Build history of the part. All positions in model axes, mm. A direction names the side the tool comes from. Round coordinates to 2 decimals unless told otherwise and drop trailing zeros. Write each loop counter-clockwise with the first axis right and the second up, starting at its lowest first coordinate (ties: lowest second). Pieces come first, ordered by that corner, then holes.
from build123d import *

# Parameters (mm, degrees)
SKETCH_1_R          = 6
EXTRUDE_1_DEPTH     = 40
CUT_EXTRUDE_START   = -5
CUT_EXTRUDE_1_DEPTH = 5
CUT_EXTRUDE_2_DEPTH = 5


with BuildPart() as part:
    # 草图1 → 凸台-拉伸1 (new body)
    with BuildSketch(Plane.XY):
        Circle(SKETCH_1_R)
    extrude(amount=EXTRUDE_1_DEPTH)

    # 草图2 → 切除-拉伸1 (cut)
    with BuildSketch(Plane.XY.offset(40).offset(CUT_EXTRUDE_START)):
        with BuildLine():
            Line((2.5, 3), (-2.5, 3))
            Line((-2.5, 3), (-2.5, 5.454356057))
            ThreePointArc((-2.5, 5.454356057), (0, 6), (2.5, 5.454356057))
            Line((2.5, 5.454356057), (2.5, 3))
        make_face()
    extrude(amount=CUT_EXTRUDE_1_DEPTH, mode=Mode.SUBTRACT)

    # 草图3 → 切除-拉伸2 (cut)
    with BuildSketch(Plane(origin=(0, 0, 0), x_dir=(-1, 0, 0), z_dir=(0, 0, -1))):
        with BuildLine():
            Line((2.5, 3), (-2.5, 3))
            Line((-2.5, 3), (-2.5, 5.454356057))
            ThreePointArc((-2.5, 5.454356057), (0, 6), (2.5, 5.454356057))
            Line((2.5, 5.454356057), (2.5, 3))
        make_face()
    extrude(amount=-CUT_EXTRUDE_2_DEPTH, mode=Mode.SUBTRACT)


solid = part.part
1) Slice it at C-C (x = 1.75). Write the cut outline in (y, z).
Results:
outline: (-5.74, 0) - (3, 0) - (3, 5) - (5.74, 5) - (5.74, 35) - (3, 35) - (3, 40) - (-5.74, 40) - close
2) Slice it at B-B (z = 12). Write the cut outline in (x, y), plus the area to 3 significant figures.
Results:
outline: circle Ø12 at (0, 0)
area: 113 mm2
3) Pin check, flat tips, straight feed: pin 1 Ø1.2 at (y, z) = (4, 38) entering from +X; pin 2 Ø1.2 at (y, z) = (3.5, 2) entering from +X; pin 3 Ø2 at (y, z) = (3.5, 14.5) entering from -X. Stop position of each tip, or through.
Results:
pin 1: stops at x = 4.94
pin 2: stops at x = 5.25
pin 3: stops at x = -5.45
4) Which spindle directions (+Z, -Z, +X, -X, +Y, -Y) get a long thin tool onto all of the face, cutting with end or side? Do faces 1 (the flat face through (0, 5, 35)), 2 (the flat face through (2.5, 4, 2)), 3 (the flat face through (0, 0, 0)). Say none if no direction does.
Results:
face 1: +Z, +Y
face 2: -Z, +Y
face 3: -Z, +X, -X, +Y, -Y
5) Mould opens along X. For faces 4 (the flat face through (0, 0, 40)), 5 (the flat face through (0, 5, 5)), 6 (the cylindrical face through (-1.301, -5.857, 19.72)) say: released by +X, released by -X, zero draft, split by the parting line, or undercut.
Results:
face 4: zero draft
face 5: undercut
face 6: split by the parting line
6) Slice it at A-A (x = 0). Write the cut outline in (y, z).
Results:
outline: (-6, 0) - (3, 0) - (3, 5) - (6, 5) - (6, 35) - (3, 35) - (3, 40) - (-6, 40) - close
7) Wall check: L1, parallel to Y at x = 0.25, z = 2.5; L2, parallel to X at y = 4, z = 24; L3, parallel to X at y = 2.5, z = 21.5. Give the ranges that are in metal, low to high.
Results:
L1: y = -5.99 to 3
L2: x = -4.47 to 4.47
L3: x = -5.45 to 5.45
8) Slice it at D-D (x = -5). Write the cut outline in (y, z), plus the area to 3 significant figures.
Results:
outline: (-3.32, 0) - (3.32, 0) - (3.32, 40) - (-3.32, 40) - close
area: 265 mm2
